Solid Edge part; units mm, degrees
sketch "Sketch1" plane through (0, 0, 0) normal (0, 0, 1) x (1, 0, 0)
  line L0 (0, 0) -> (0, 12.7)
  line L1 (0, 12.7) -> (76.2, 12.7)
  line L2 (76.2, 12.7) -> (76.2, 0)
  line L3 (76.2, 0) -> (0, 0)
  dimension "D1" = 76.2
extrude "Protrusion1" add sketch "Sketch1" along normal blind 9.525
hole "Hole_1" at (38.1, 6.35, 9.525) direction (0, 0, -1) diameter 6.35 end up to next
hole "Hole1" at (66.675, 6.35, 9.525) direction (0, 0, -1) diameter 6.35 end up to next
hole "Hole2" at (9.525, 6.35, 9.525) direction (0, 0, -1) diameter 6.35 end up to next
chamfer "Chamfer_1" distance 3.175 angle 45 1 edges at (38.1, 0, 9.525)
Can you work these out from the model? Positions are in its coordinate system, mm. Round coordinates to 2 decimals unless told otherwise and drop trailing zeros. Order: outer loops, then holes, each group sorted by start corner. A loop starts at its lowest first (then second) coordinate and runs counter-clockwise, first axis right, second up. Notation, with made-up numbers: (83, 35) -> (107, 35) arc R7 cw to (107, 45) -> close; hole circle Ø3 at (-35.5, 19.5). An arc over 180 degrees is marked (long way). Return JSON: item names as keys, results as strings. Group by question number.
1. If we section it at D-D, the plane z = 4.75: Write out the boundary of the cut face in (x, y) (3 decimals).
2. Will this pin go through, and if not, where does the flat tip stop? pin 1 (5 mm diameter, centred on x = 38.1, y = 6.35, fed in from +Z).
3. I need wall thicknesses on line 1 (X direction, y = 6.35, z = 5.75) (3 decimals); line 2 (X direction, y = 8, z = 3.25); line 3 (Y direction, x = 38.1, z = 6.5) (3 decimals). Which ranges of each line are inside material? Lowest first, please. Write a range as [from, to].
4. If we section it at B-B, the plane y = 6.35: Write out the boundary of the cut face in (x, z) (3 decimals), then the cut area to 3 significant figures.
5. If we section it at C-C, the plane x = 57: Write out the boundary of the cut face in (y, z) (3 decimals).
6. We'd pull the mould along Y, two halves only. Please class faces 1 (the face through (38.63, 1.61, 7.96)), 2 (the face through (39, 2, 0)), 3 (the face through (38, 12.7, 5)), 4 (the face through (63.576, 7.038, 4.829)): released by +Y, released by -Y, zero draft, split by the parting line, or undercut.
Output values:
{
 "1": {"outline": "(0, 0) -> (76.2, 0) -> (76.2, 12.7) -> (0, 12.7) -> close; hole circle Ø6.35 at (9.525, 6.35); hole circle Ø6.35 at (38.1, 6.35); hole circle Ø6.35 at (66.675, 6.35)"},
 "2": {"pin 1": "through"},
 "3": {"line 1": "[0, 6.35], [12.7, 34.925], [41.275, 63.5], [69.85, 76.2]", "line 2": "[0, 6.81], [12.24, 35.39], [40.81, 63.96], [69.39, 76.2]", "line 3": "[0.15, 3.175], [9.525, 12.7]"},
 "4": {"outline": "(0, 0) -> (6.35, 0) -> (6.35, 9.525) -> (0, 9.525) -> close; (12.7, 0) -> (34.925, 0) -> (34.925, 9.525) -> (12.7, 9.525) -> close; (41.275, 0) -> (63.5, 0) -> (63.5, 9.525) -> (41.275, 9.525) -> close; (69.85, 0) -> (76.2, 0) -> (76.2, 9.525) -> (69.85, 9.525) -> close", "area": "544 mm²"},
 "5": {"outline": "(0, 0) -> (12.7, 0) -> (12.7, 9.525) -> (3.175, 9.525) -> (0, 6.35) -> close"},
 "6": {"face 1": "released by -Y", "face 2": "zero draft", "face 3": "released by +Y", "face 4": "undercut"}
}
